```python
from build123d import *

# Parameters (mm, degrees)
F0_W        = 6.35
F0_H        = 2.54
F1_DEPTH    = 76.2
F2_R        = 1.27
F3_T1_DEPTH = 82.55


# Not quite as in the source:
# - a fillet or chamfer that OpenCascade refuses, or shapes differently, is made with other operations: its cross-section is extruded or revolved along the edge and cut away or added


with BuildPart() as f1:
    # F0 (on Front) → F1 (new body)
    with BuildSketch(Plane.XZ):
        Polygon((-43.1055540526, 26.5985474133), (-40.5655540526, 26.5985474133), (-34.2155540526, 26.5985474133), (-34.2155540526, 27.8685474133), (-43.1055540526, 27.8685474133), align=None)
        Polygon((-40.5655540526, 20.2485474133), (-40.5655540526, 26.5985474133), (-43.1055540526, 26.5985474133), (-43.1055540526, 17.7085474133), (-40.5655540526, 17.7085474133), align=None)
        with Locations((-37.3905540526, 18.9785474133)):
            Rectangle(F0_W, F0_H)
    extrude(amount=F1_DEPTH)

    # F2
    f2_edges = [f1.edges().sort_by_distance(p)[0] for p in [
        (-43.105554, -38.1, 27.868547),
    ]]
    fillet(f2_edges, radius=F2_R)

    # F3: fillet of radius 1.27 on 5 edges, made by hand

    # F3_s2 → F3_t1 (cut)
    with BuildSketch(Plane.XZ.offset(-3.175)):
        with BuildLine():
            ThreePointArc((-43.1055540526, 18.9785474133), (-42.7335796647, 18.0805218012), (-41.8355540526, 17.7085474133))
            Line((-41.8355540526, 17.7085474133), (-43.1055540526, 17.7085474133))
            Line((-43.1055540526, 17.7085474133), (-43.1055540526, 18.9785474133))
        make_face()
        with BuildLine():
            ThreePointArc((-34.2155540526, 27.8685474133), (-34.5875284405, 26.9705218012), (-35.4855540526, 26.5985474133))
            Line((-35.4855540526, 26.5985474133), (-34.2155540526, 26.5985474133))
            Line((-34.2155540526, 26.5985474133), (-34.2155540526, 27.8685474133))
        make_face()
        with BuildLine():
            ThreePointArc((-34.2155540526, 18.9785474133), (-34.5875284405, 19.8765730255), (-35.4855540526, 20.2485474133))
            Line((-35.4855540526, 20.2485474133), (-34.2155540526, 20.2485474133))
            Line((-34.2155540526, 20.2485474133), (-34.2155540526, 18.9785474133))
        make_face()
        with BuildLine():
            ThreePointArc((-35.4855540526, 17.7085474133), (-34.5875284405, 18.0805218012), (-34.2155540526, 18.9785474133))
            Line((-34.2155540526, 18.9785474133), (-34.2155540526, 17.7085474133))
            Line((-34.2155540526, 17.7085474133), (-35.4855540526, 17.7085474133))
        make_face()
        with BuildLine():
            ThreePointArc((-35.4855540526, 27.8685474133), (-34.5875284405, 27.4965730255), (-34.2155540526, 26.5985474133))
            Line((-34.2155540526, 26.5985474133), (-34.2155540526, 27.8685474133))
            Line((-34.2155540526, 27.8685474133), (-35.4855540526, 27.8685474133))
        make_face()
    extrude(amount=F3_T1_DEPTH, mode=Mode.SUBTRACT)


solid = f1.part
```
Build history of the part. All positions in model axes, mm. A direction names the side the tool comes from. Coordinates: 2 decimals unless noted, no trailing zeros. Order: outer loops, then holes, each group sorted by start corner. A loop starts at its lowest first (then second) coordinate and runs counter-clockwise, first axis right, second up.
Item 1: Drill centre lines: L1, parallel to Z at x = -37, y = -71.5; L2, parallel to X at y = -54.5, z = 23; L3, parallel to Z at x = -35, y = -33.5. Where is each one in solid material? Low to high.
Filled in:
L1: z = 17.71 to 20.25, 26.6 to 27.87
L2: x = -43.11 to -40.57
L3: z = 17.81 to 20.15, 26.7 to 27.77
Item 2: Mould opens along Z. For faces 1 (the flat face through (-39, -38, 17.709)), 2 (the flat face through (-41, 0, 23)), 3 (the flat face through (-38, -38, 20.249)) say: released by +Z, released by -Z, zero draft, split by the parting line, or undercut.
Filled in:
face 1: released by -Z
face 2: zero draft
face 3: undercut
Item 3: Tool access for faces 4 (the flat face through (-41, -76.2, 23)), 5 (the flat face through (-38, -38, 26.599)): list every direction of +Z, -Z, +X, -X, +Y, -Y with a clear straight run to the whole face (end or side of a thin tool).
Filled in:
face 4: +Z, -Z, +X, -X, -Y
face 5: +X, +Y, -Y
Item 4: Saw through at B-B on y = -64.5. List the corners of the cut face in (x, z).
Filled in:
outline: (-43.11, 18.98) arc R1.27 ccw to (-41.84, 17.71) - (-35.49, 17.71) arc R1.27 ccw to (-35.49, 20.25) - (-40.57, 20.25) - (-40.57, 26.6) - (-35.49, 26.6) arc R1.27 ccw to (-34.39, 27.23) arc R1.27 ccw to (-35.49, 27.87) - (-41.84, 27.87) arc R1.27 ccw to (-43.11, 26.6) - close
Item 5: Drop flat-ended pins along their axis: pin 1 Ø1.5 at (x, y) = (-42, -49.5) entering from +Z; pin 2 Ø6 at (y, z) = (-58, 25.5) entering from +X; pin 3 Ø1 at (y, z) = (-43, 25) entering from +X; pin 4 Ø4 at (y, z) = (-21.5, 22) entering from +X. Give the stop position or say it passes through.
Filled in:
pin 1: stops at z = 27.87
pin 2: stops at x = -34.39
pin 3: stops at x = -40.57
pin 4: stops at x = -34.73
Item 6: Saw through at C-C on z = 25.25. List the corners of the cut face in (x, y).
Filled in:
outline: (-43.11, -76.2) - (-40.57, -76.2) - (-40.57, 0) - (-43.11, 0) - close
Item 7: Saw through at A-A on x = -37.5. List the corners of the cut face in (y, z).
Filled in:
outline: (-76.2, 17.71) - (0, 17.71) - (0, 20.25) - (-76.2, 20.25) - close; (-76.2, 26.6) - (0, 26.6) - (0, 27.87) - (-76.2, 27.87) - close
